```python
from build123d import *

# Parameters (mm, degrees)
SKETCH_1_R          = 6.7
SKETCH_1_R_2        = 1.650002274
SKETCH_1_R_3        = 1.65
EXTRUDE_1_DEPTH     = 3
FILLET_1_R          = 5
FILLET_2_R          = 20
CUT_EXTRUDE_1_DEPTH = 202.075524607


with BuildPart() as part:
    # 草图1 → 凸台-拉伸1 (new body)
    with BuildSketch(Plane(origin=(0, 0, 0), x_dir=(1, 0, 0), z_dir=(0, 1, 0))):
        with BuildLine():
            Line((0, 0), (50, 0))
            Line((50, 0), (50, 200))
            ThreePointArc((50, 200), (23.223304703, 176.776695297), (0, 150))
            Line((0, 150), (0, 0))
        make_face()
        with Locations(Location((10, 80, 0), (0, 0, 270))):
            Circle(SKETCH_1_R, mode=Mode.SUBTRACT)
        with Locations(Location((10, 144, 0), (0, 0, 270))):
            Circle(SKETCH_1_R, mode=Mode.SUBTRACT)
        with Locations(Location((10, 30, 0), (0, 0, 270))):
            Circle(SKETCH_1_R_2, mode=Mode.SUBTRACT)
        with Locations(Location((45.5, 30, 0), (0, 0, 270))):
            Circle(SKETCH_1_R_3, mode=Mode.SUBTRACT)
        with Locations(Location((45.5, 115, 0), (0, 0, 270))):
            Circle(SKETCH_1_R_3, mode=Mode.SUBTRACT)
        with BuildLine():
            Line((8.35, 5), (8.35, 17.2))
            ThreePointArc((8.35, 17.2), (10, 18.85), (11.65, 17.2))
            Line((11.65, 17.2), (11.65, 5))
            ThreePointArc((11.65, 5), (10, 3.35), (8.35, 5))
        make_face(mode=Mode.SUBTRACT)
        with BuildLine():
            Line((8.35, 42.8), (8.35, 55))
            ThreePointArc((8.35, 55), (10, 56.65), (11.65, 55))
            Line((11.65, 55), (11.65, 42.8))
            ThreePointArc((11.65, 42.8), (10, 41.15), (8.35, 42.8))
        make_face(mode=Mode.SUBTRACT)
        with BuildLine():
            Line((43.85, 5), (43.85, 17.2))
            ThreePointArc((43.85, 17.2), (45.5, 18.85), (47.15, 17.2))
            Line((47.15, 17.2), (47.15, 5))
            ThreePointArc((47.15, 5), (45.5, 3.35), (43.85, 5))
        make_face(mode=Mode.SUBTRACT)
        with BuildLine():
            Line((43.85, 42.8), (43.85, 55))
            ThreePointArc((43.85, 55), (45.5, 56.65), (47.15, 55))
            Line((47.15, 55), (47.15, 42.8))
            ThreePointArc((47.15, 42.8), (45.5, 41.15), (43.85, 42.8))
        make_face(mode=Mode.SUBTRACT)
        with BuildLine():
            Line((43.85, 90), (43.85, 102.2))
            ThreePointArc((43.85, 102.2), (45.5, 103.85), (47.15, 102.2))
            Line((47.15, 102.2), (47.15, 90))
            ThreePointArc((47.15, 90), (45.5, 88.35), (43.85, 90))
        make_face(mode=Mode.SUBTRACT)
        with BuildLine():
            Line((43.85, 127.8), (43.85, 140))
            ThreePointArc((43.85, 140), (45.5, 141.65), (47.15, 140))
            Line((47.15, 140), (47.15, 127.8))
            ThreePointArc((47.15, 127.8), (45.5, 126.15), (43.85, 127.8))
        make_face(mode=Mode.SUBTRACT)
    extrude(amount=EXTRUDE_1_DEPTH)

    # 圆角1
    fillet_1_edges = [part.edges().sort_by_distance(p)[0] for p in [
        (50, 1.5, -200),
        (50, 1.5, 0),
        (0, 1.5, 0),
    ]]
    fillet(fillet_1_edges, radius=FILLET_1_R)

    # 圆角2
    fillet_2_edges = [part.edges().sort_by_distance(p)[0] for p in [
        (0, 1.5, -150),
    ]]
    fillet(fillet_2_edges, radius=FILLET_2_R)

    # 草图2 → 切除-拉伸1 (cut, through all)
    with BuildSketch(Plane(origin=(0, 3, 0), x_dir=(1, 0, 0), z_dir=(0, 1, 0))):
        with BuildLine():
            Line((36.85, 141), (36.85, 20))
            ThreePointArc((36.85, 20), (29.925, 13.075), (23, 20))
            Line((23, 20), (23, 141))
            ThreePointArc((23, 141), (29.925, 147.925), (36.85, 141))
        make_face()
    extrude(amount=-CUT_EXTRUDE_1_DEPTH, mode=Mode.SUBTRACT)


solid = part.part
```
Verification items for the finished model (mm, model axes). A direction names the side the tool comes from. Give positions to 0.01 mm unless a question says otherwise; leave off trailing zeros. Order: outer loops, then holes, each group sorted by start corner. A loop starts at its lowest first (then second) coordinate and runs counter-clockwise, first axis right, second up. Notation, with made-up numbers: (29, -38) -> (50, -38) arc R15 ccw to (50, -30) -> close; hole circle Ø8 at (62.25, 44.25). An arc over 180 degrees is marked (long way). One line per item, written item: value.
(1) Tool access check on faces 4 (the face through (30.077, 1.521, -13.077)), 5 (the face through (48, 2, -1)). Record the directions out of +Z, -Z, +X, -X, +Y, -Y that give a thin tool (end or side, any length) a straight path to the whole face; none if there is none.
Final values:
face 4: +Y, -Y
face 5: +Z, +X, +Y, -Y
(2) Draft check along Z on faces 1 (the face through (1.087, 1.521, -149.683)), 2 (the face through (12.01, 1.48, -137.61)), 3 (the face through (19, 3, -99)). Enter one of: pulls with the +Z half, pulls with the -Z half, needs draft (parallel to the pull), parting line crosses it, or undercut.
Final values:
face 1: pulls with the -Z half
face 2: undercut
face 3: needs draft
(3) Scan lines: line 1 along X through (y, z) = (1.25, -115); line 2 along X through (y, z) = (0.55, -44). Record each from-to range of solid material in increasing order. Write a range as [from, to].
Final values:
line 1: [0, 23], [36.85, 43.85], [47.15, 50]
line 2: [0, 8.35], [11.65, 23], [36.85, 43.85], [47.15, 50]
(4) Sectioned sample at C-C on z = -65. Record the cut outline in (x, y).
Final values:
outline: (0, 0) -> (23, 0) -> (23, 3) -> (0, 3) -> close; (36.85, 0) -> (50, 0) -> (50, 3) -> (36.85, 3) -> close
(5) Sectioned sample at D-D on z = -30. Record the cut outline in (x, y).
Final values:
outline: (0, 0) -> (8.35, 0) -> (8.35, 3) -> (0, 3) -> close; (11.65, 0) -> (23, 0) -> (23, 3) -> (11.65, 3) -> close; (36.85, 0) -> (43.85, 0) -> (43.85, 3) -> (36.85, 3) -> close; (47.15, 0) -> (50, 0) -> (50, 3) -> (47.15, 3) -> close
(6) Sectioned sample at B-B on x = 14. Record the cut outline in (y, z).
Final values:
outline: (0, -167.04) -> (3, -167.04) -> (3, -149.37) -> (0, -149.37) -> close; (0, -138.63) -> (3, -138.63) -> (3, -85.37) -> (0, -85.37) -> close; (0, -74.63) -> (3, -74.63) -> (3, 0) -> (0, 0) -> close
(7) Sectioned sample at A-A on z = -115. Record the cut outline in (x, y), then the cut area to 4 significant figures.
Final values:
outline: (0, 0) -> (23, 0) -> (23, 3) -> (0, 3) -> close; (36.85, 0) -> (43.85, 0) -> (43.85, 3) -> (36.85, 3) -> close; (47.15, 0) -> (50, 0) -> (50, 3) -> (47.15, 3) -> close
area: 98.55 mm^2
(8) Gauge pin test, flat ends, axial feed: pin 1 (3 mm diameter, centred on x = 45.5, z = -115, fed in from -Y); pin 2 (4 mm diameter, centred on x = 45.5, z = -30, fed in from -Y). Record the tip position at first contact, or that the pin passes through.
Final values:
pin 1: through
pin 2: y = 0
